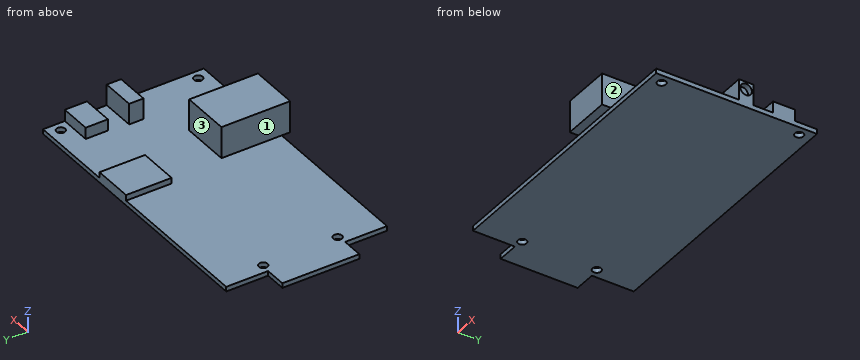
```python
from build123d import *

# Parameters (mm, degrees)
F0_R     = 1.5
F0_W     = 14.2
F0_H     = 15.9
F0_W_2   = 11.8
F0_H_2   = 5
F1_DEPTH = 1.65
F2_W     = 14
F2_H     = 15.9
F3_DEPTH = 2
F2_W_2   = 11
F2_H_2   = 7.74
F4_DEPTH = 4
F2_W_3   = 17
F2_H_3   = 21
F2_H_4   = 3
F5_DEPTH = 11
F6_W     = 11.8
F6_H     = 5
F7_DEPTH = 7.3
F8_R     = 2
F9_DEPTH = 2


with BuildPart() as f1:
    # F0 (on Top) → F1 (new body)
    with BuildSketch(Plane.XY):
        Polygon((4.39, 28.06), (-48.25, 28.06), (-48.25, 13.44), (-55.75, 13.44), (-55.75, 0), (-55.75, -13.44), (-48.25, -13.44), (-48.25, -28.06), (48.25, -28.06), (48.25, 0), (48.25, 0.81), (36.45, 0.81), (36.45, 5.81), (48.25, 5.81), (48.25, 28.06), (18.59, 28.06), (18.59, 12.16), (4.39, 12.16), align=None)
        with Locations((-45, -13)):
            Circle(F0_R, mode=Mode.SUBTRACT)
        with Locations((45, -24)):
            Circle(F0_R, mode=Mode.SUBTRACT)
        with Locations((-45, 13)):
            Circle(F0_R, mode=Mode.SUBTRACT)
        with Locations((45, 24)):
            Circle(F0_R, mode=Mode.SUBTRACT)
        with Locations((11.49, 20.11)):
            Rectangle(F0_W, F0_H)
        with Locations((42.35, 3.31)):
            Rectangle(F0_W_2, F0_H_2)
    extrude(amount=F1_DEPTH)

    # F2 (on face) → F3 (join)
    with BuildSketch(Plane.XY.offset(1.65)):
        with Locations((11.5, 20.11)):
            Rectangle(F2_W, F2_H)
    extrude(amount=F3_DEPTH)

    # F2 (on face) → F4 (join)
    with BuildSketch(Plane.XY.offset(1.65)):
        with Locations((42.75, 16.59)):
            Rectangle(F2_W_2, F2_H_2)
    extrude(amount=F4_DEPTH)

    # F2 (on face) → F5 (join)
    with BuildSketch(Plane.XY.offset(1.65)):
        with Locations((15.75, -17.56)):
            Rectangle(F2_W_3, F2_H_3)
        with Locations((15.75, -29.56)):
            Rectangle(F2_W_3, F2_H_4)
    extrude(amount=F5_DEPTH)

    # F6 (on face) → F7 (join)
    with BuildSketch(Plane.XY.offset(1.65)):
        with Locations((42.35, 3.31)):
            Rectangle(F6_W, F6_H)
    extrude(amount=F7_DEPTH)

    # F8 (on face) → F9 (cut)
    with BuildSketch(Plane.YZ.offset(48.25)):
        with Locations((3.31, 6.25)):
            Circle(F8_R)
    extrude(amount=-F9_DEPTH, mode=Mode.SUBTRACT)


solid = f1.part
```
Could you check a few things on this model? Use its own coordinates, in mm. Face numbers are marked on the shaded views. A direction names the side the tool comes from. Coordinates: 2 decimals unless noted, no trailing zeros. Write each loop counter-clockwise with the first axis right and the second up, starting at its lowest first coordinate (ties: lowest second). Pieces come first, ordered by that corner, then holes. Notation, with made-up numbers: (84, 58.25) - (110, 58.25) arc R17 ccw to (110, 71.25) - close; hole circle Ø9 at (27, 68.5). An arc over 180 degrees is marked (long way). Use a Markdown table: item, result.
Q1. I'm going to push flat-ended pins straight in: pin 1 Ø2.5 at (y, z) = (3.31, 6.25) entering from -X; pin 2 Ø0.8 at (y, z) = (-23, 0.5) entering from -X; pin 3 Ø4 at (x, y) = (45, -24) entering from -Z; pin 4 Ø3.5 at (x, y) = (-45, 13) entering from +Z. Where does each tip first touch, or does it pass through?
Geometry check:
| item | result |
|---|---|
| pin 1 | stops at x = 36.45 |
| pin 2 | stops at x = -48.25 |
| pin 3 | stops at z = 0 |
| pin 4 | stops at z = 1.65 |
Q2. Imagine slicing it at A-A (x = 45). List the corners of the cut face in (y, z) for me, and give its area (3 significant figures).
Geometry check:
| item | result |
|---|---|
| outline | (-28.06, 0) - (-25.5, 0) - (-25.5, 1.65) - (-28.06, 1.65) - close; (-22.5, 0) - (22.5, 0) - (22.5, 1.65) - (20.46, 1.65) - (20.46, 5.65) - (12.72, 5.65) - (12.72, 1.65) - (5.81, 1.65) - (5.81, 8.95) - (0.81, 8.95) - (0.81, 1.65) - (-22.5, 1.65) - close; (25.5, 0) - (28.06, 0) - (28.06, 1.65) - (25.5, 1.65) - close |
| area | 150 mm2 |
Q3. Imagine slicing it at D-D (x = -45). List the corners of the cut face in (y, z) for me.
Geometry check:
| item | result |
|---|---|
| outline | (-28.06, 0) - (-14.5, 0) - (-14.5, 1.65) - (-28.06, 1.65) - close; (-11.5, 0) - (11.5, 0) - (11.5, 1.65) - (-11.5, 1.65) - close; (14.5, 0) - (28.06, 0) - (28.06, 1.65) - (14.5, 1.65) - close |
Q4. Imagine slicing it at B-B (y = -24). List the corners of the cut face in (x, z) for me, and give its area (3 significant figures).
Geometry check:
| item | result |
|---|---|
| outline | (-48.25, 0) - (43.5, 0) - (43.5, 1.65) - (24.25, 1.65) - (24.25, 12.65) - (7.25, 12.65) - (7.25, 1.65) - (-48.25, 1.65) - close; (46.5, 0) - (48.25, 0) - (48.25, 1.65) - (46.5, 1.65) - close |
| area | 341 mm2 |
Q5. Which directions (+Z, -Z, +X, -X, +Y, -Y) give clear straight access to the entire face, cutting with the end or side of a thin tool? Please do the marked faces 1, 2 and 3.
Geometry check:
| item | result |
|---|---|
| face 1 | +Z, -X, -Y |
| face 2 | +Z, +X, +Y, -Y |
| face 3 | +Z, +X, -X |
Q6. Imagine slicing it at C-C (y = 19). List the corners of the cut face in (x, z) for me, and give its area (3 significant figures).
Geometry check:
| item | result |
|---|---|
| outline | (-48.25, 0) - (48.25, 0) - (48.25, 5.65) - (37.25, 5.65) - (37.25, 1.65) - (18.5, 1.65) - (18.5, 3.65) - (4.5, 3.65) - (4.5, 1.65) - (-48.25, 1.65) - close |
| area | 231 mm2 |
Q7. Please list where these lines run through material, in increasing order: L1, parallel to Y at x = -45, z = 1.15; L2, parallel to Y at x = 45, z = 0.7; L3, parallel to X at y = 2, z = 6.
Geometry check:
| item | result |
|---|---|
| L1 | y = -28.06 to -14.5, -11.5 to 11.5, 14.5 to 28.06 |
| L2 | y = -28.06 to -25.5, -22.5 to 22.5, 25.5 to 28.06 |
| L3 | x = 36.45 to 46.25 |
